Read the model definition and answer for the solid it produces. Units are mm, in the model's axes. A direction names the side the tool comes from. Round coordinates to 2 decimals unless told otherwise and drop trailing zeros. Order: outer loops, then holes, each group sorted by start corner. A loop starts at its lowest first (then second) coordinate and runs counter-clockwise, first axis right, second up. Notation, with made-up numbers: (85.5, 85) -> (128.5, 85) arc R15 ccw to (128.5, 92) -> close; hole circle Ø11 at (35, -25). An arc over 180 degrees is marked (long way). One line per item, written item: value. Start each with the question number.
1. Section B-B (y = -24.5) is taken. Give the vertices of the cut face in (x, z), then the cut area to 3 significant figures.
2. For faces 5 (the face through (-16, -6, -6)), 6 (the face through (5.15, 3.373, 14.632)), 7 (the face through (17.521, -2.018, 15.368)), determine the directions among +Z, -Z, +X, -X, +Y, -Y from which every point of the face is accessible in a straight line to the end or side of a thin tool.
3. Section D-D (x = 11) is taken. Give the vertices of the cut face in (y, z).
4. Section A-A (z = 0) is taken. Give the vertices of the cut face in (x, y), then the cut area to 3 significant figures.
5. Consider line 1 (Z direction, x = 12.5, y = 0.5); line 2 (X direction, y = 0, z = 13); line 3 (X direction, y = -11.5, z = -15). Determine where each line is inside the solid, lowest interval first.
6. Section C-C (z = 25) is taken. Give the vertices of the cut face in (x, y), then the cut area to 3 significant figures.
7. Flat-ended cylindrical pins translate along their axes: pin 1 Ø13 at (x, y) = (3, 0) entering from +Z; pin 2 Ø6.5 at (y, z) = (0, 23) entering from +X; pin 3 Ø10 at (y, z) = (-19, -21.5) entering from +X; pin 4 Ø22.5 at (y, z) = (0, 0) entering from +X. Find the tip coordinate at first contact, or state that the pin passes through.
8. The mould has two halves that part along X. Classify faces 1 (the face through (-11, 13, -13)), 2 (the face through (4.846, -3.549, -14.711)), 3 (the face through (-19, 0, 0)), 4 (the face through (-17.479, -7.493, 0.33)): released by +X, released by -X, zero draft, split by the parting line, or undercut.
from build123d import *

# Parameters (mm, degrees)
CUT_EXTRUDE1_REACH      = 53.386
SKETCH2_R               = 3.5
CUT_EXTRUDE2_DEPTH      = 46.84212037
CUT_EXTRUDE2_DEPTH_BACK = 46.84212037
SKETCH3_R               = 4


# Read off the part's stored shape, not the designer's step: Revolve1
with BuildPart() as part:
    # Revolve1 outline → Revolve1 (revolve)
    with BuildSketch(Plane.YX):
        Polygon((0, -9), (0, -19), (7.5, -19), (7.5, -16), (29.5, -16), (29.5, -11), (17.5, -11), (17.5, 16), (15.5, 16), (15.5, 19), (12.5, 19), (12.5, -9), align=None)
    revolve(axis=Axis((0, 0, 0), (1, 0, 0)))

    # Sketch2 → Cut-Extrude1 (cut, up to next)
    with BuildSketch(Plane(origin=(-11, 0, 0), x_dir=(0, 0, -1), z_dir=(1, 0, 0)), mode=Mode.PRIVATE) as cut_extrude1_sk1:
        with Locations((0, 23)):
            Circle(SKETCH2_R)
    cut_extrude1_tool1 = extrude(cut_extrude1_sk1.sketch, amount=-CUT_EXTRUDE1_REACH, mode=Mode.PRIVATE) & part.part
    # Sketch2 → Cut-Extrude1 (cut, up to next)
    with BuildSketch(Plane(origin=(-11, 0, 0), x_dir=(0, 0, -1), z_dir=(1, 0, 0)), mode=Mode.PRIVATE) as cut_extrude1_sk2:
        with Locations((23, 0)):
            Circle(SKETCH2_R)
    cut_extrude1_tool2 = extrude(cut_extrude1_sk2.sketch, amount=-CUT_EXTRUDE1_REACH, mode=Mode.PRIVATE) & part.part
    # Sketch2 → Cut-Extrude1 (cut, up to next)
    with BuildSketch(Plane(origin=(-11, 0, 0), x_dir=(0, 0, -1), z_dir=(1, 0, 0)), mode=Mode.PRIVATE) as cut_extrude1_sk3:
        with Locations((0, -23)):
            Circle(SKETCH2_R)
    cut_extrude1_tool3 = extrude(cut_extrude1_sk3.sketch, amount=-CUT_EXTRUDE1_REACH, mode=Mode.PRIVATE) & part.part
    # Sketch2 → Cut-Extrude1 (cut, up to next)
    with BuildSketch(Plane(origin=(-11, 0, 0), x_dir=(0, 0, -1), z_dir=(1, 0, 0)), mode=Mode.PRIVATE) as cut_extrude1_sk4:
        with Locations((-23, 0)):
            Circle(SKETCH2_R)
    cut_extrude1_tool4 = extrude(cut_extrude1_sk4.sketch, amount=-CUT_EXTRUDE1_REACH, mode=Mode.PRIVATE) & part.part
    add(cut_extrude1_tool1.solids().sort_by_distance((-11, 23, 0))[0], mode=Mode.SUBTRACT)
    add(cut_extrude1_tool2.solids().sort_by_distance((-11, 0, -23))[0], mode=Mode.SUBTRACT)
    add(cut_extrude1_tool3.solids().sort_by_distance((-11, -23, 0))[0], mode=Mode.SUBTRACT)
    add(cut_extrude1_tool4.solids().sort_by_distance((-11, 0, 23))[0], mode=Mode.SUBTRACT)

    # Sketch3 → Cut-Extrude2 (cut, two sides: drawn at the far end of the back side and taken through both)
    with BuildSketch(Plane.XY.offset(-CUT_EXTRUDE2_DEPTH_BACK)):
        with Locations((3, 0)):
            Circle(SKETCH3_R)
    extrude(amount=CUT_EXTRUDE2_DEPTH + CUT_EXTRUDE2_DEPTH_BACK, mode=Mode.SUBTRACT)


solid = part.part
Answer:
1. outline: (-16, -16.43) -> (-11, -16.43) -> (-11, -3.16) -> (-16, -3.16) -> close; (-16, 3.16) -> (-11, 3.16) -> (-11, 16.43) -> (-16, 16.43) -> close
1. area: 133 mm^2
2. face 5: -X
2. face 6: +Z, -Z
2. face 7: +X
3. outline: circle Ø35 at (0, 0); hole circle Ø25 at (0, 0)
4. outline: (-19, -7.5) -> (-16, -7.5) -> (-16, -19.5) -> (-11, -19.5) -> (-11, -17.5) -> (16, -17.5) -> (16, -15.5) -> (19, -15.5) -> (19, -12.5) -> (-9, -12.5) -> (-9, 12.5) -> (19, 12.5) -> (19, 15.5) -> (16, 15.5) -> (16, 17.5) -> (-11, 17.5) -> (-11, 19.5) -> (-16, 19.5) -> (-16, 7.5) -> (-19, 7.5) -> close; (-16, -29.5) -> (-11, -29.5) -> (-11, -26.5) -> (-16, -26.5) -> close; (-16, 26.5) -> (-11, 26.5) -> (-11, 29.5) -> (-16, 29.5) -> close
4. area: 608 mm^2
5. line 1: -17.49 to -12.49, 12.49 to 17.49
5. line 2: -16 to -1, 7 to 19
5. line 3: -16 to -11
6. outline: (-16, -15.66) -> (-11, -15.66) -> (-11, -2.87) -> (-16, -2.87) -> close; (-16, 2.87) -> (-11, 2.87) -> (-11, 15.66) -> (-16, 15.66) -> close
6. area: 128 mm^2
7. pin 1: z = 17.5
7. pin 2: through
7. pin 3: x = -11
7. pin 4: x = -9
8. face 1: released by +X
8. face 2: undercut
8. face 3: released by -X
8. face 4: zero draft
